```python
from build123d import *

# Parameters (mm, degrees)
ESQUISSE1_R                  = 2.5
ESQUISSE1_R_2                = 1.5
BOSS_EXTRU_1_DEPTH           = 5
BOSS_EXTRU_2_START           = -15
ESQUISSE2_R                  = 3.5
ESQUISSE2_R_2                = 2.5
BOSS_EXTRU_2_DEPTH           = 10
ESQUISSE3_R                  = 3.5
BOSS_EXTRU_3_DEPTH           = 3
CONG_1_R                     = 0.5
ENL_V_MAT_EXTRU_1_DEPTH      = 26.124689053
ENL_V_MAT_EXTRU_1_DEPTH_BACK = 26.124689053
ESQUISSE4_R                  = 1.5
ESQUISSE5_R                  = 3.5
ESQUISSE5_R_2                = 2.5
BOSS_EXTRU_4_DEPTH           = 6
CONG_2_R                     = 1
CONG_3_R                     = 1


with BuildPart() as part:
    # Esquisse1 → Boss.-Extru.1 (new body)
    with BuildSketch(Plane.XY):
        with BuildLine():
            Line((-17.5, 5), (17.5, 5))
            ThreePointArc((17.5, 5), (22.5, 0), (17.5, -5))
            Line((17.5, -5), (-17.5, -5))
            ThreePointArc((-17.5, -5), (-22.5, 0), (-17.5, 5))
        make_face()
        with Locations((-17.5, 0)):
            Circle(ESQUISSE1_R, mode=Mode.SUBTRACT)
        with Locations((17.5, 0)):
            Circle(ESQUISSE1_R_2, mode=Mode.SUBTRACT)
    extrude(amount=BOSS_EXTRU_1_DEPTH)

    # Esquisse2 → Boss.-Extru.2 (add)
    with BuildSketch(Plane.XY.offset(5).offset(BOSS_EXTRU_2_START)):
        with Locations((-17.5, 0)):
            Circle(ESQUISSE2_R)
        with Locations((-17.5, 0)):
            Circle(ESQUISSE2_R_2, mode=Mode.SUBTRACT)
    extrude(amount=BOSS_EXTRU_2_DEPTH)

    # Esquisse3 → Boss.-Extru.3 (add)
    with BuildSketch(Plane(origin=(0, 0, -10), x_dir=(-1, 0, 0), z_dir=(0, 0, -1))):
        with Locations(Location((17.5, 0, 0), (0, 0, 180))):
            Circle(ESQUISSE3_R)
    extrude(amount=-BOSS_EXTRU_3_DEPTH)

    # Congé1
    cong_1_edges = [part.edges().sort_by_distance(p)[0] for p in [
        (-21, 0, -10),
    ]]
    fillet(cong_1_edges, radius=CONG_1_R)

    # Esquisse4 → Enlèv. mat.-Extru.1 (cut, two sides: drawn at the far end of the back side and taken through both)
    with BuildSketch(Plane(origin=(0, 0, 0), x_dir=(1, 0, 0), z_dir=(0, 1, 0)).offset(-ENL_V_MAT_EXTRU_1_DEPTH_BACK)):
        with Locations(Location((-17.5, 4.75, 0), (0, 0, 270))):
            Circle(ESQUISSE4_R)
    extrude(amount=ENL_V_MAT_EXTRU_1_DEPTH + ENL_V_MAT_EXTRU_1_DEPTH_BACK, mode=Mode.SUBTRACT)

    # Esquisse5 → Boss.-Extru.4 (add)
    with BuildSketch(Plane.XY.offset(5)):
        with Locations((-17.5, 0)):
            Circle(ESQUISSE5_R)
        with Locations(Location((-17.5, 0, 0), (0, 0, 180))):
            Circle(ESQUISSE5_R_2, mode=Mode.SUBTRACT)
    extrude(amount=BOSS_EXTRU_4_DEPTH)

    # Congé2
    cong_2_edges = [part.edges().sort_by_distance(p)[0] for p in [
        (-21, 0, 5),
    ]]
    fillet(cong_2_edges, radius=CONG_2_R)

    # Congé3
    cong_3_edges = [part.edges().sort_by_distance(p)[0] for p in [
        (-21, 0, 0),
    ]]
    fillet(cong_3_edges, radius=CONG_3_R)


solid = part.part
```
Model file for the job. Use its own axes, mm. A direction names the side the tool comes from. Give positions to 0.01 mm unless a question says otherwise; leave off trailing zeros. Write each loop counter-clockwise with the first axis right and the second up, starting at its lowest first coordinate (ties: lowest second). Pieces come first, ordered by that corner, then holes. Notation, with made-up numbers: (63, 35.25) - (90, 35.25) arc R23 ccw to (90, 74.25) - close; hole circle Ø4 at (75.25, -38). An arc over 180 degrees is marked (long way). One line per question, with ' | ' between items. Start each with the question number.
(1) Pin check, flat tips, straight feed: P1, Ø6, axis at x = 18, y = -3.5, coming from the -Z side; P2, Ø2.5, axis at x = -18, y = -1, coming from the +Z side; P3, Ø6, axis at x = 10.5, z = -4.5, coming from the +Y side; P4, Ø2, axis at y = 1, z = -7, coming from the -X side. Stop position of each tip, or through.
(2) Slice it at A-A on z = 1. Write the cut outline in (x, y).
(3) Slice it at B-B on z = -4.75. Write the cut outline in (x, y), plus the area to 3 significant figures.
(4) Two-plate mould, pull along X, no slides. Class faces 1 (the face through (-20, 1, 11)), 2 (the face through (-16.235, -2.762, -3.944)), 3 (the face through (-14.16, 1.05, 8.46)), 4 (the face through (-16.235, 2.741, -3.944)): +X half, -X half, draft (parallel to the pull), parting line (faces both ways), or undercut.
(5) 3-axis set-ups, long thin cutter, end or side, ignore diameter. For faces 5 (the face through (-18, 0, -7)), 6 (the face through (-15.885, -3.105, -5.31)), 7 (the face through (16, 0, 2)): which of +Z, -Z, +X, -X, +Y, -Y reach the whole face in a straight line?
(6) Slice it at C-C on x = 15.5. Write the cut outline in (y, z), plus the area to 3 significant figures.
(7) Wall check: line 1 along Y through (x, z) = (-17.5, 2.25); line 2 along Z through (x, y) = (-17.5, 2.95); line 3 along Y through (x, z) = (17.5, 2.3). Give the ranges that are in metal, low to high. Write a range as from..to.
(8) Slice it at D-D on z = 8.5. Write the cut outline in (x, y).
Results below:
1) P1: z = 0 | P2: z = -7 | P3: through | P4: x = -21
2) outline: (-17.5, -5) - (17.5, -5) arc R5 ccw to (17.5, 5) - (-17.5, 5) arc R5 ccw to start; hole circle Ø5 at (-17.5, 0); hole circle Ø3 at (17.5, 0)
3) outline: (-19, -3.16) - (-19, -2) arc R2.5 cw to (-19, 2) - (-19, 3.16) arc R3.5 ccw to start; (-16, -3.16) arc R3.5 ccw to (-16, 3.16) - (-16, 2) arc R2.5 cw to (-16, -2) - close | area: 12.6 mm^2
4) face 1: draft | face 2: undercut | face 3: parting line | face 4: undercut
5) face 5: +Z | face 6: -Z | face 7: +Z, -Z
6) outline: (-5, 0) - (5, 0) - (5, 5) - (-5, 5) - close | area: 50.0 mm^2
7) line 1: -5..-2.5, 2.5..5 | line 2: -10..-6.25, -3.25..11 | line 3: -5..-1.5, 1.5..5
8) outline: circle Ø7 at (-17.5, 0); hole circle Ø5 at (-17.5, 0)
